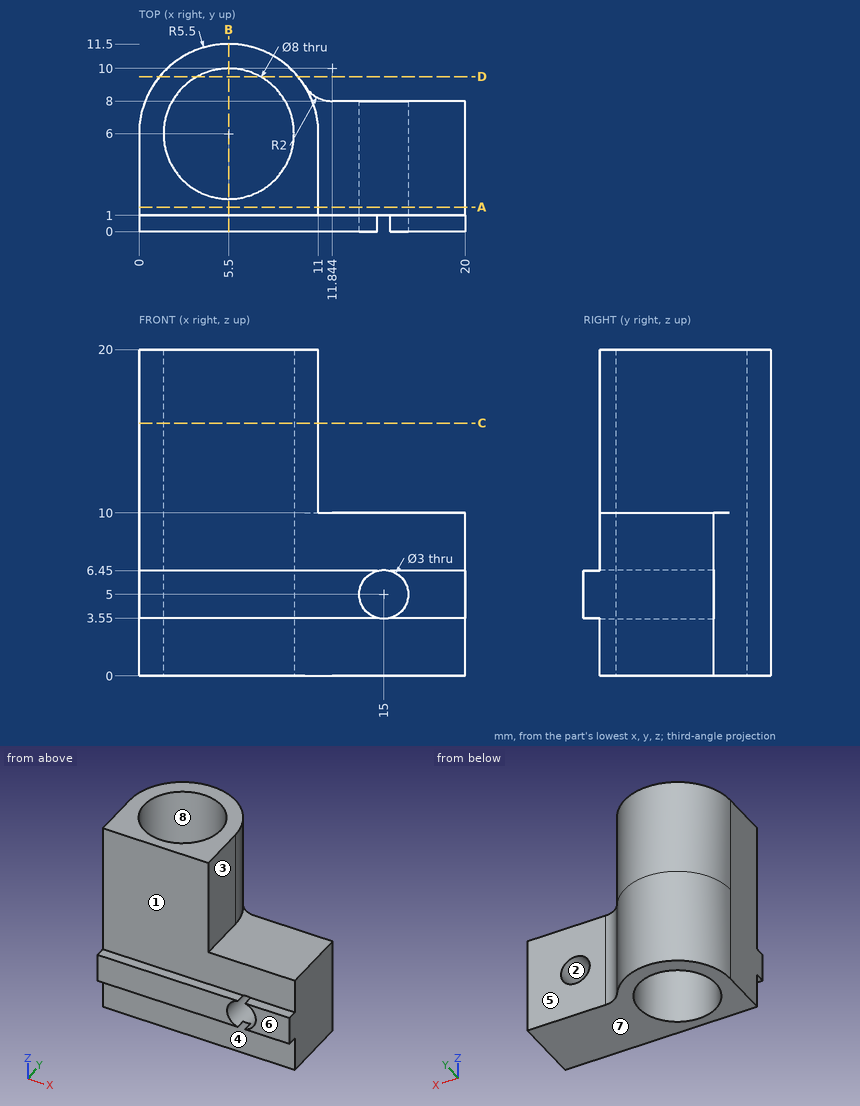
Here's the drawing with two shaded views (mm, measured from the low corner). I have some questions. A direction names the side the tool comes from. Give positions to 0.01 mm unless a question says otherwise; leave off trailing zeros. Loops run counter-clockwise (first coordinate to the right, second up) from the corner with the lowest first, then second, coordinate; pieces in that order, holes last. Notation, with made-up numbers: M 28,-7 L 56,-7 A23 ccw 56,21 Z; hole C -19,59 d7. An arc over 180 degrees is marked long. One line per item, written item: value.
1) Imagine slicing it at B-B on x = 5.5. Write out the boundary of the cut face in (y, z).
Geometry check:
outline: M 0,3.55 L 1,3.55 L 1,0 L 2,0 L 2,20 L 1,20 L 1,6.45 L 0,6.45 Z; M 10,0 L 11.5,0 L 11.5,20 L 10,20 Z
2) Imagine slicing it at A-A on y = 1.5. Write out the boundary of the cut face in (x, z), and give its area (3 significant figures).
Geometry check:
outline: M 0,0 L 20,0 L 20,10 L 11,10 L 11,20 L 0,20 Z; hole C 15,5 d3
area: 303 mm²
3) I'm going to push flat-ended pins straight in: pin 1 (6.5 mm diameter, centred on x = 16.5, y = 5, fed in from +Z); pin 2 (6 mm diameter, centred on x = 5.5, y = 6, fed in from +Z); pin 3 (0.8 mm diameter, centred on x = 7.5, y = 0.5, fed in from -Z); pin 4 (0.5 mm diameter, centred on x = 18.5, y = 0.5, fed in from +Z). Where does each tip first touch, or does it pass through?
Geometry check:
pin 1: stops at z = 10
pin 2: passes through
pin 3: stops at z = 3.55
pin 4: stops at z = 6.45
4) On a 3-axis mill with a long thin cutter (end or side, diameter ignored), from which of +Z, -Z, +X, -X, +Y, -Y can I reach the whole of each face in a straight line? I mean the marked faces 1, 2, 3 and 4. Say none if no direction works.
Geometry check:
face 1: +Z, +X, -X, -Y
face 2: +Y, -Y
face 3: +Z, +X, +Y, -Y
face 4: -Z, +X, -X, -Y
5) Imagine slicing it at D-D on y = 9.5. Write out the boundary of the cut face in (x, z).
Geometry check:
outline: M 1.26,0 L 3.56,0 L 3.56,20 L 1.26,20 Z; M 7.44,0 L 9.74,0 L 9.74,20 L 7.44,20 Z
6) Thinking about a two-plate mould opening in Y: for the marked faces 5, 6, 7 and 8, which applies, +Y half, -Y half, draft (parallel to the pull), parting line (faces both ways), or undercut?
Geometry check:
face 5: +Y half
face 6: -Y half
face 7: draft
face 8: undercut
7) Please list where these lines run through material, in increasing order: line 1 (Y direction, x = 5.5, z = 10.5); line 2 (Z direction, x = 15, y = 3.25); line 3 (Y direction, x = 12, z = 3).
Geometry check:
line 1: y = 1 to 2, 10 to 11.5
line 2: z = 0 to 3.5, 6.5 to 10
line 3: y = 1 to 8
8) Imagine slicing it at C-C on z = 15.5. Write out the boundary of the cut face in (x, y).
Geometry check:
outline: M 0,1 L 11,1 L 11,6 A5.5 ccw 0,6 Z; hole C 5.5,6 d8
